Autodesk Inventor part; units mm, degrees
ref_plane "YZ Plane" through (0, 0, 0) normal (1, 0, 0) x (0, 1, 0)
ref_plane "XZ Plane" through (0, 0, 0) normal (0, 1, 0) x (-1, 0, 0)
ref_plane "XY Plane" through (0, 0, 0) normal (0, 0, 1) x (1, 0, 0)
sketch "Sketch1" plane through (0, 0, 0) normal (0, 1, 0) x (-1, 0, 0)
  line L0 (0, 0) -> (-254, 0)
  line L1 (-254, 0) -> (-254, 88.9)
  line L2 (-254, 88.9) -> (0, 88.9)
  line L3 (0, 88.9) -> (0, 0)
  line L4 (0, -76.2) -> (-254, -76.2)
  line L5 (-254, -76.2) -> (-254, -165.1)
  line L6 (-254, -165.1) -> (0, -165.1)
  line L7 (0, -165.1) -> (0, -76.2)
  dimension "d0" = 88.9
  dimension "d1" = 254
  dimension "d2" = 254
  dimension "d3" = 88.9
  dimension "d4" = 76.2
extrude "Extrusion1" add sketch "Sketch1" along normal blind 25.4
sketch "Sketch2" plane through (0, 25.4, 0) normal (0, 1, 0) x (1, 0, 0)
  line L0 (0, -88.9) -> (25.4, -88.9)
  line L1 (25.4, -88.9) -> (25.4, -63.5)
  line L2 (25.4, -63.5) -> (0, -63.5)
  line L3 (0, -63.5) -> (0, -88.9)
  line L4 (0, 165.1) -> (114.3, 165.1)
  line L5 (114.3, 165.1) -> (114.3, 139.7)
  line L6 (114.3, 139.7) -> (0, 139.7)
  line L7 (0, 139.7) -> (0, 165.1)
  point P0 (25.4, 139.7)
  dimension "d7" = 25.4
  dimension "d17" = 114.3
  dimension "d18" = 25.4
extrude "Extrusion2" add sketch "Sketch2" along normal blind 31.75
sketch "Sketch3" plane through (0, 0, 88.9) normal (0, 0, 1) x (1, 0, 0)
  circle A0 centre (12.7, 44.45) radius 12.7
  line L0 (25.4, 57.15) -> (0, 57.15)
  point P0 (0, 0)
  dimension "d13" = 12.7
  dimension "d14" = 25.4
extrude "Extrusion3" add sketch "Sketch3" against normal blind 242.8875
sketch "Sketch4" plane through (0, 57.15, 0) normal (0, 1, 0) x (1, 0, 0)
  line L0 (0, 165.1) -> (0, 76.2)
  line L1 (0, 165.1) -> (197.3764, 165.1)
  line L2 (197.3764, 165.1) -> (197.3764, 139.7)
  line L3 (197.3764, 139.7) -> (0, 139.7)
  line L4 (0, 139.7) -> (0, 165.1)
  point P0 (0, 0)
extrude "Extrusion4" add sketch "Sketch4" along normal blind 165.1
chamfer "Chamfer1" distance 80.9625 angle 45 1 edges at (197.3764, 57.15, -152.4)
properties part number "handbase"
Input: part model. Units: mm. Frame: model coordinates. A direction names the side the tool comes from. Round coordinates to 2 decimals unless told otherwise and drop trailing zeros. Order: outer loops, then holes, each group sorted by start corner. A loop starts at its lowest first (then second) coordinate and runs counter-clockwise, first axis right, second up. Notation, with made-up numbers: (15.25, -6.75) - (23.25, -6.75) arc R14 cw to (23.25, 13.25) - close; hole circle Ø8 at (-29, 31). An arc over 180 degrees is marked (long way). Answer as a JSON object with one key per item and string values. Group by question number.
(1) Pin query (flat end, axial travel): P1, Ø12.5, axis at y = 48.5, z = -157.5, coming from the +X side; P2, Ø20.5, axis at y = 196, z = -148.5, coming from the +X side; P3, Ø20.5, axis at x = 8.5, z = 80, coming from the +Y side. Return the tip coordinate at first contact, or that it passes through.
(2) Cut plane A-A (x = 107.5). Return loops of the section in (y, z), then the cut area to 3 significant figures.
(3) Draft query along Z for faces 6 (the face through (125, 13, 0)), 7 (the face through (114.3, 41, -153)), 8 (the face through (23, 54, 63.5)), 9 (the face through (97, 110, -165.1)). Return one class per face: released by +Z, released by -Z, zero draft, split by the parting line, or undercut.
(4) Cut plane B-B (z = 10.5). Return loops of the section in (x, y).
(5) Cut plane D-D (z = -23). Return loops of the section in (x, y), then the cut area to 3 significant figures.
(6) Material intervals for probe 1 along Z at (x, y) = (154, 15.5); probe 2 along Z at (x, y) = (92.5, 47.5); probe 3 along Y at (x, z) = (208, 28), sorted ascending. Write a range as from..to.
(7) Cut plane C-C (y = 170.5). Return loops of the section in (x, z).
(8) Reachability of faces 1 (the face through (13, 31, 63.5)), 2 (the face through (129, 0, 45)), 3 (the face through (13, 57.15, 76)), 4 (the face through (25.4, 41, 76)), 5 (the face through (3, 55, 63.5)) from +Z, -Z, +X, -X, +Y, -Y: full face, straight path, thin tool, end or side. Return the list, or none.
Here are the results:
{
 "1": {"P1": "stops at x = 114.3", "P2": "stops at x = 197.38", "P3": "stops at y = 57.15"},
 "2": {"outline": "(0, -165.1) - (222.25, -165.1) - (222.25, -139.7) - (25.4, -139.7) - (25.4, -76.2) - (0, -76.2) - close; (0, 0) - (25.4, 0) - (25.4, 88.9) - (0, 88.9) - close", "area": "9,520 mm^2"},
 "3": {"face 6": "undercut", "face 7": "zero draft", "face 8": "undercut", "face 9": "released by -Z"},
 "4": {"outline": "(0, 0) - (254, 0) - (254, 25.4) - (0, 25.4) - close; circle Ø25.4 at (12.7, 44.45)"},
 "5": {"outline": "circle Ø25.4 at (12.7, 44.45)", "area": "507 mm^2"},
 "6": {"probe 1": "z = -165.1..-76.2, 0..88.9", "probe 2": "z = -165.1..-139.7", "probe 3": "y = 0..25.4"},
 "7": {"outline": "(0, -165.1) - (197.38, -165.1) - (197.38, -139.7) - (0, -139.7) - close"},
 "8": {"face 1": "none", "face 2": "+Z, -Z, +X, -X, -Y", "face 3": "+Z, +X, -X, +Y", "face 4": "+Z, +X, +Y", "face 5": "-X, +Y"}
}
